Drawing for the job (mm, zero at the part's lowest x, y, z). Give positions to 0.01 mm unless a question says otherwise; leave off trailing zeros. Order: outer loops, then holes, each group sorted by start corner. A loop starts at its lowest first (then second) coordinate and runs counter-clockwise, first axis right, second up. Notation, with made-up numbers: (49, 87.25) - (97, 87.25) arc R31 ccw to (97, 125.25) - close; hole circle Ø3 at (-25, -4). An arc over 180 degrees is marked (long way). Use CSV: the item, a comma, the result in double quotes. Start each with the question number.
(1) Band-saw the part on C-C, the plane y = 0.6. Give the cut face in (x, z), then the cut area to 3 significant figures.
(2) Band-saw the part on B-B, the plane z = 28.5. Give the cut face in (x, y), then the cut area to 3 significant figures.
(3) Pull direction Z, two halves, no side cores. Call the marked faces 1, 2 and 3: +Z half, -Z half, draft (parallel to the pull), parting line (faces both ways), or undercut.
(4) Drop flat-ended pins along their axis: pin 1 Ø1.3 at (x, y) = (10.5, 1.5) entering from -Z; pin 2 Ø4.5 at (x, z) = (7, 7) entering from +Y. Give the stop position or say it passes through.
(5) Band-saw the part on A-A, the plane x = 7. Give the cut face in (y, z).
(6) Band-saw the part on D-D, the plane x = 13.25. Give the cut face in (y, z).
(7) Probe L1, parallel to X at y = 0.9, z = 28.5; L2, parallel to Z at x = 7, y = 1.35; L3, parallel to Z at x = 7.75, y = 1.05. List the from-to ranges inside material, lowest first.
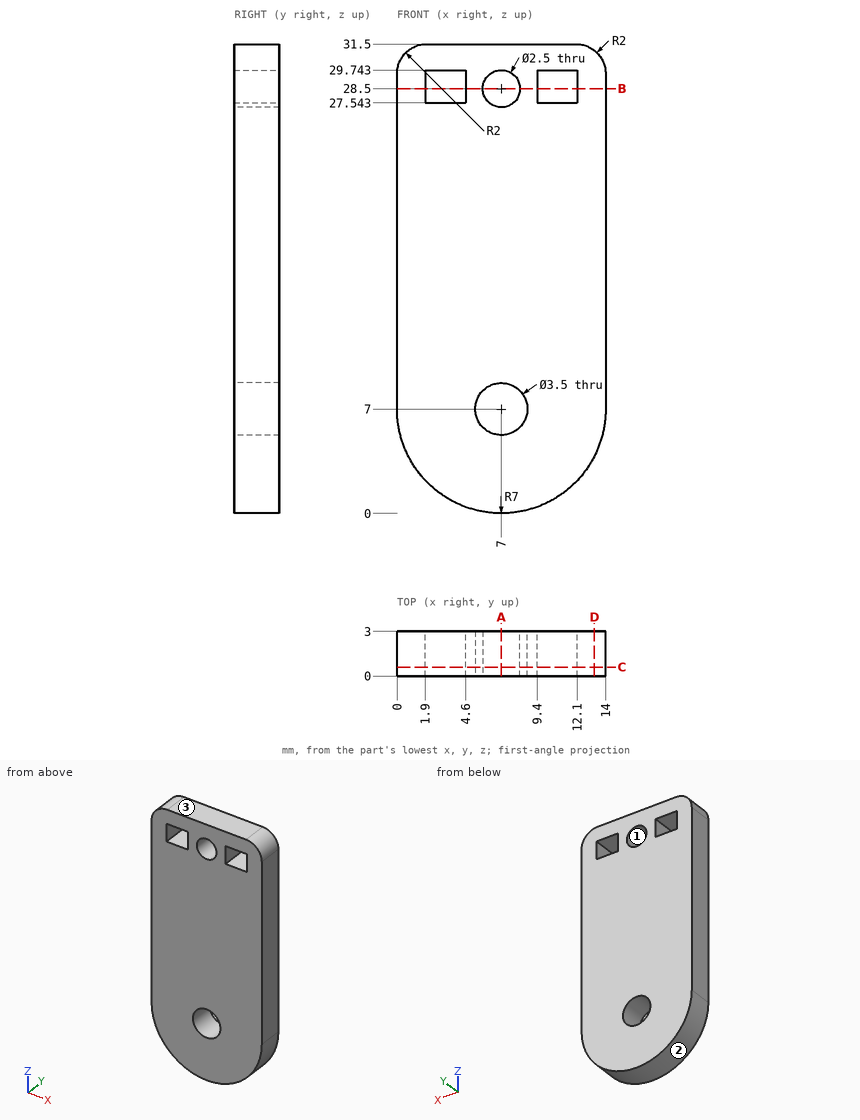
Answer block:
1,outline,"(0, 7) arc R7 ccw to (14, 7) - (14, 29.5) arc R2 ccw to (12, 31.5) - (2, 31.5) arc R2 ccw to (0, 29.5) - close; hole (1.9, 27.54) - (4.6, 27.54) - (4.6, 29.74) - (1.9, 29.74) - close; hole circle Ø3.5 at (7, 7); hole circle Ø2.5 at (7, 28.5); hole (9.4, 27.54) - (12.1, 27.54) - (12.1, 29.74) - (9.4, 29.74) - close"
1,area,"392 mm2"
2,outline,"(0, 0) - (1.9, 0) - (1.9, 3) - (0, 3) - close; (4.6, 0) - (5.75, 0) - (5.75, 3) - (4.6, 3) - close; (8.25, 0) - (9.4, 0) - (9.4, 3) - (8.25, 3) - close; (12.1, 0) - (14, 0) - (14, 3) - (12.1, 3) - close"
2,area,"18.3 mm2"
3,face 1,"undercut"
3,face 2,"-Z half"
3,face 3,"+Z half"
4,pin 1,"stops at z = 0.61"
4,pin 2,"stops at y = 3"
5,outline,"(0, 0) - (3, 0) - (3, 5.25) - (0, 5.25) - close; (0, 8.75) - (3, 8.75) - (3, 27.25) - (0, 27.25) - close; (0, 29.75) - (3, 29.75) - (3, 31.5) - (0, 31.5) - close"
6,outline,"(0, 3.85) - (3, 3.85) - (3, 31.06) - (0, 31.06) - close"
7,L1,"x = 0 to 1.9, 4.6 to 5.75, 8.25 to 9.4, 12.1 to 14"
7,L2,"z = 0 to 5.25, 8.75 to 27.25, 29.75 to 31.5"
7,L3,"z = 0.04 to 5.42, 8.58 to 27.5, 29.5 to 31.5"
